Verification items for the finished model (mm, model axes). A direction names the side the tool comes from. Coordinates: 2 decimals unless noted, no trailing zeros. Order: outer loops, then holes, each group sorted by start corner. A loop starts at its lowest first (then second) coordinate and runs counter-clockwise, first axis right, second up. Notation, with made-up numbers: (42, 11) -> (93, 11) arc R21 ccw to (93, 39) -> close; hole circle Ø8 at (46.25, -10). An arc over 180 degrees is marked (long way). Write item = value, one per line. Start each with the question number.
1. Cross-section at C-C on x = 57.5. Record the cut outline in (y, z), plus the area to 3 significant figures.
2. Thickness scan on line 1 along Z through (x, y) = (64, 18); line 2 along Z through (x, y) = (55, 18); line 3 along Y through (x, z) = (44.5, -4.5). Record the ranges inside material, lowest first. Write a range as from..to.
3. Release check for a two-part mould opening along Y. For faces 1 (the flat face through (44.238, 5.293, 1.686)), 2 (the flat face through (59.287, 23, 27.2)), 3 (the flat face through (44.232, 36.186, -3.233)), 4 (the flat face through (44.24, 44.69, 1.73)) record: +Y half, -Y half, draft (parallel to the pull), parting line (faces both ways), or undercut.
4. Cross-section at B-B on x = 67.5. Record the cut outline in (y, z).
5. Set-up check for faces 5 (the flat face through (44.24, 5.31, -1.73)), 6 (the flat face through (44.2, 10.84, 4.93)), 7 (the flat face through (52, 30, 0)), 8 (the flat face through (67, 5, 25)), 9 (the flat face through (67, 45, 25)): record each of +Z, -Z, +X, -X, +Y, -Y from which the full face is reachable in a straight line by a thin tool's end or side.
6. Cross-section at A-A on x = 45.5. Record the cut outline in (y, z).
7. Go/stop test with flat-tipped pins: P1, Ø5.5, axis at x = 65.5, z = -25.5, coming from the -Y side; P2, Ø1.5, axis at y = 41, z = 13.5, coming from the -X side; P3, Ø1.5, axis at x = 64.5, y = 13.5, coming from the -Z side; P4, Ø10, axis at x = 63.5, z = 5.5, coming from the +Y side. Record where each tip stops, or that it passes through.
from build123d import *

# Parameters (mm, degrees)
BOSS_EXTRUDE1_DEPTH      = 50
SHELL1_T                 = -5
BOSS_EXTRUDE2_DEPTH      = 7.5
BOSS_EXTRUDE2_DEPTH_BACK = 5
SKETCH4_W                = 20
SKETCH4_H                = 10
CUT_EXTRUDE1_DEPTH       = 10
FILLET1_RADIUS           = 2.5
FILLET1_LENGTH           = 50
FILLET2_RADIUS           = 2.5
FILLET2_LENGTH           = 50
SKETCH7_W                = 16
SKETCH7_H                = 5
CUT_EXTRUDE3_DEPTH       = 10


with BuildPart() as part:
    # Sketch2 → Boss-Extrude1 (new body)
    with BuildSketch(Plane(origin=(0, 0, 0), x_dir=(1, 0, 0), z_dir=(0, 1, 0))):
        with BuildLine():
            Line((46.545206992, 27.5), (49.2865347, 27.5))
            Line((49.2865347, 27.5), (59.2865347, 27.5))
            Line((59.2865347, 27.5), (59.2865347, 27))
            Line((59.2865347, 27), (75.2865347, 27))
            Line((75.2865347, 27), (75.2865347, -27))
            Line((75.2865347, -27), (59.2865347, -27))
            Line((59.2865347, -27), (59.2865347, -27.5))
            Line((59.2865347, -27.5), (49.2865347, -27.5))
            Line((49.2865347, -27.5), (46.545206992, -27.5))
            add(Edge.make_bspline(
                [(46.545206992, -27.5), (52.189315716, 0), (46.545206992, 27.5)],
                knots=[4.377296144, 4.377296144, 4.377296144, 5.047481816, 5.047481816, 5.047481816], degree=2, weights=[1, 0.944379784, 1]))
        make_face()
    extrude(amount=BOSS_EXTRUDE1_DEPTH)

    # Shell1
    shell1_openings = [part.faces().sort_by_distance(p)[0] for p in [
        (61.762813671, 50, 0),
        (61.762813671, 0, 0),
        (75.2865347, 25, 0),
    ]]
    offset(amount=SHELL1_T, openings=shell1_openings, kind=Kind.INTERSECTION)

    # Sketch3 → Boss-Extrude2 (add, two sides: drawn at the far end of the back side and taken through both)
    with BuildSketch(Plane.ZY.offset(-46.545206992).offset(-BOSS_EXTRUDE2_DEPTH_BACK)):
        Polygon((-5.240052605, 40.923962655), (-4.608024926, 37.339555569), (-1.819851171, 35), (1.819851171, 35), (4.608024926, 37.339555569), (5.240052605, 40.923962655), (3.420201433, 44.076037345), (0, 45.320888862), (-3.420201433, 44.076037345), align=None)
        Polygon((0, 4.679111138), (3.420201433, 5.923962655), (5.240052605, 9.076037345), (4.608024926, 12.660444431), (1.819851171, 15), (-1.819851171, 15), (-4.608024926, 12.660444431), (-5.240052605, 9.076037345), (-3.420201433, 5.923962655), align=None)
    extrude(amount=BOSS_EXTRUDE2_DEPTH + BOSS_EXTRUDE2_DEPTH_BACK)

    # Sketch4 → Cut-Extrude1 (cut)
    with BuildSketch(Plane.ZY.offset(-46.545206992)):
        with Locations((0, 25)):
            Rectangle(SKETCH4_W, SKETCH4_H)
    extrude(amount=-CUT_EXTRUDE1_DEPTH, mode=Mode.SUBTRACT)

    # Fillet1: full round fillet: the end face becomes a half cylinder, R = half its width
    fillet1_face = Plane((75.2865347, 25, -24.5), x_dir=(0, 1, 0), z_dir=(1, 0, 0))  # on the end face: x along it, z out of the body
    fillet1_slab = fillet1_face.offset(-FILLET1_RADIUS / 2) * Box(FILLET1_LENGTH, 2 * FILLET1_RADIUS, FILLET1_RADIUS, mode=Mode.PRIVATE)  # the body's end, R deep
    fillet1_round = Plane((72.7865347, 25, -24.5), x_dir=(1, 0, 0), z_dir=(0, 1, 0)) * Cylinder(FILLET1_RADIUS, FILLET1_LENGTH, mode=Mode.PRIVATE)  # its axis R under the face
    add(fillet1_slab - fillet1_round, mode=Mode.SUBTRACT)

    # Fillet2: full round fillet: the end face becomes a half cylinder, R = half its width
    fillet2_face = Plane((75.2865347, 25, 24.5), x_dir=(0, -1, 0), z_dir=(1, 0, 0))  # on the end face: x along it, z out of the body
    fillet2_slab = fillet2_face.offset(-FILLET2_RADIUS / 2) * Box(FILLET2_LENGTH, 2 * FILLET2_RADIUS, FILLET2_RADIUS, mode=Mode.PRIVATE)  # the body's end, R deep
    fillet2_round = Plane((72.7865347, 25, 24.5), x_dir=(1, 0, 0), z_dir=(0, -1, 0)) * Cylinder(FILLET2_RADIUS, FILLET2_LENGTH, mode=Mode.PRIVATE)  # its axis R under the face
    add(fillet2_slab - fillet2_round, mode=Mode.SUBTRACT)

    # Sketch7 → Cut-Extrude3 (cut)
    with BuildSketch(Plane.XY.offset(27)):
        with Locations((67.2865347, 47.5)):
            Rectangle(SKETCH7_W, SKETCH7_H)
        with Locations((67.2865347, 2.5)):
            Rectangle(SKETCH7_W, SKETCH7_H)
    cut_extrude3 = extrude(amount=-CUT_EXTRUDE3_DEPTH, mode=Mode.SUBTRACT)

    # Mirror2: Cut-Extrude3 across plane
    add(cut_extrude3.mirror(Plane.XY), mode=Mode.SUBTRACT)


solid = part.part
Worked out:
q1.outline = (0, -27.5) -> (50, -27.5) -> (50, -22) -> (0, -22) -> close; (0, 22) -> (50, 22) -> (50, 27.5) -> (0, 27.5) -> close
q1.area = 550 mm²
q2.line_1 = -27..-22, 22..27
q2.line_2 = -27.5..-22, 22..27.5
q2.line_3 = 7.79..12.75, 37.25..42.21
q3.face_1 = -Y half
q3.face_2 = draft
q3.face_3 = undercut
q3.face_4 = +Y half
q4.outline = (5, -27) -> (45, -27) -> (45, -22) -> (5, -22) -> close; (5, 22) -> (45, 22) -> (45, 27) -> (5, 27) -> close
q5.face_5 = -X, -Y
q5.face_6 = -X
q5.face_7 = +X, -X
q5.face_8 = +Z, -Z, +X, -Y
q5.face_9 = +Z, -Z, +X, +Y
q6.outline = (4.68, 0) -> (5.92, -3.42) -> (9.08, -5.24) -> (12.66, -4.61) -> (15, -1.82) -> (15, 1.82) -> (12.66, 4.61) -> (9.08, 5.24) -> (5.92, 3.42) -> close; (35, -1.82) -> (37.34, -4.61) -> (40.92, -5.24) -> (44.08, -3.42) -> (45.32, 0) -> (44.08, 3.42) -> (40.92, 5.24) -> (37.34, 4.61) -> (35, 1.82) -> close
q7.P1 = 5
q7.P2 = 48.57
q7.P3 = -27
q7.P4 = through
